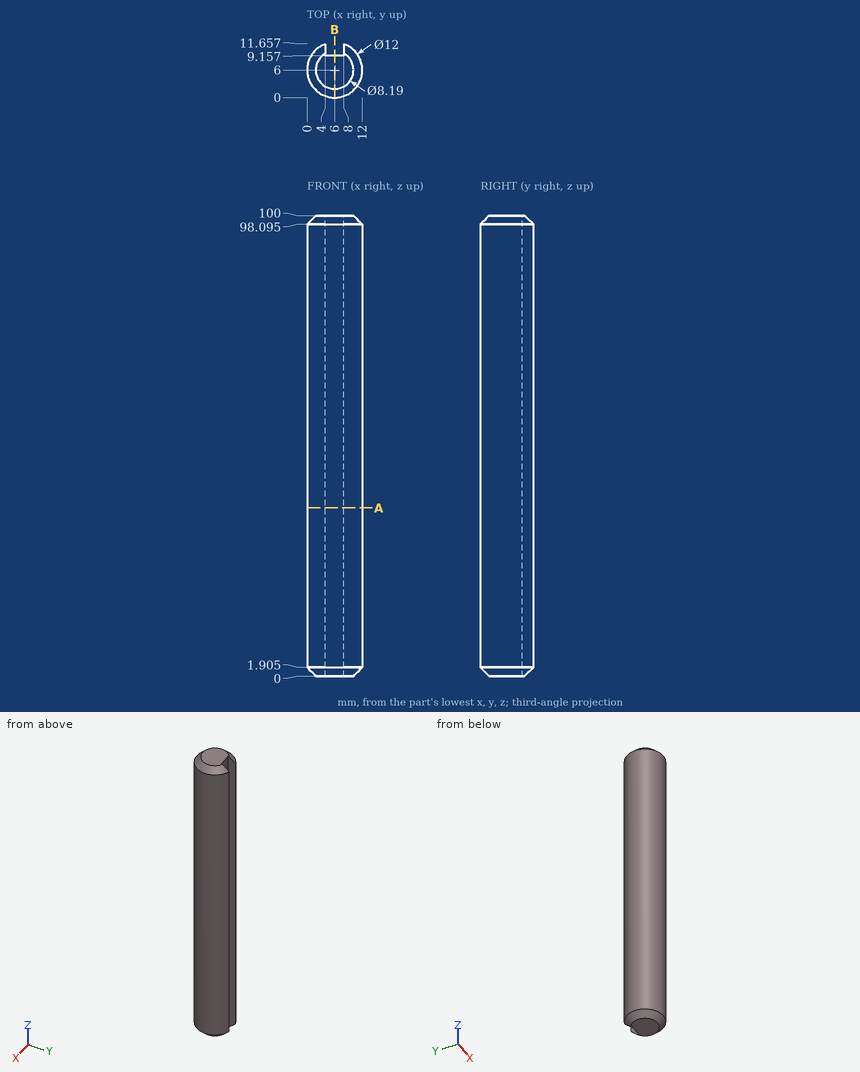
Geometry check sheet. Reference: drawing and pictorial views, mm from the part's lowest x, y, z. Round coordinates to 2 decimals unless told otherwise and drop trailing zeros. Loops run counter-clockwise (first coordinate to the right, second up) from the corner with the lowest first, then second, coordinate; pieces in that order, holes last. Notation, with made-up numbers: (8.25, 71) - (59.25, 71) arc R35 cw to (59.25, 106) - close; hole circle Ø3 at (80.25, 57.5). An arc over 180 degrees is marked (long way). Write item = value, one per line. Start each with the question number.
Q1. Depth check by flat-ended pin: P1, Ø3, axis at x = 2, z = 21.5, coming from the +Y side; P2, Ø0.8, axis at y = 10, z = 58, coming from the +X side; P3, Ø0.7, axis at y = 10.5, z = 64.5, coming from the -X side. Enter the tip coordinate at first touch or a pass-through.
Q2. Section check B-B (x = 6). Record the boundary of the cut face in (y, z) (3 decimals), plus the area to 3 significant figures.
Q3. Thickness scan on L1, parallel to X at y = 6.25, z = 64 (1 decimal); L2, parallel to X at y = 9.75, z = 14; L3, parallel to X at y = 10.25, z = 30 (1 decimal). Record the ranges inside material, lowest first.
Q4. Section check A-A (z = 36.5). Record the boundary of the cut face in (x, y).
Derived:
q1.P1 = 11.45
q1.P2 = 10.8
q1.P3 = 1.67
q2.outline = (0, 1.905) - (1.905, 0) - (9.157, 0) - (9.157, 100) - (1.905, 100) - (0, 98.095) - close
q2.area = 912 mm^2
q3.L1 = 0 to 12
q3.L2 = 1.32 to 4, 8 to 10.68
q3.L3 = 1.8 to 4, 8 to 10.2
q4.outline = (4, 9.16) - (4, 11.66) arc R6 ccw (long way) to (8, 11.66) - (8, 9.16) - close
